```python
from build123d import *

# Parameters (mm, degrees)
BASE_FLANGE1_DEPTH           = 3.175
SKETCH8_W                    = 12.7
SKETCH8_H                    = 3.175
CUT_EXTRUDE2_DEPTH           = 309.926847379
SKETCH11_R                   = 3.175
CUT_EXTRUDE4_DEPTH           = 309.926847379
SKETCH21_R                   = 2.5527
CUT_EXTRUDE5_DEPTH           = 309.926847379
SKETCH23_W                   = 25.4
SKETCH23_H                   = 3.175
TAB1_DEPTH                   = 3.175
CSK_FOR_M3_SFHCS1_AT_2_COUNT = 2
CSK_FOR_M3_SFHCS1_AT_2_PITCH = 16
CSK_FOR_M3_SFHCS1_AT_3_COUNT = 2
CSK_FOR_M3_SFHCS1_AT_3_PITCH = 27.712812921
CSK_FOR_M3_SFHCS1_AT_4_COUNT = 2
CSK_FOR_M3_SFHCS1_AT_4_PITCH = 32
CSK_FOR_M3_SFHCS1_AT_5_COUNT = 2
CSK_FOR_M3_SFHCS1_AT_5_PITCH = 27.712812921
CSK_FOR_M3_SFHCS1_AT_6_COUNT = 2
CSK_FOR_M3_SFHCS1_AT_6_PITCH = 16


# Sheet-metal steps are written as plain solids
with BuildPart() as part:
    # Sketch1 → Base-Flange1 (new body)
    with BuildSketch(Plane(origin=(0, 0, 0), x_dir=(0, 0, -1), z_dir=(1, 0, 0))):
        with BuildLine():
            Line((0, -80.9625), (0, 80.9625))
            Line((0, 80.9625), (-110.597916699, 80.9625))
            ThreePointArc((-110.597916699, 80.9625), (-137.538685062, 85.883926782), (-160.999479175, 100.0125))
            ThreePointArc((-160.999479175, 100.0125), (-201.559524406, 89.942756121), (-177.8, 55.5625))
            Line((-177.8, 55.5625), (-25.4, 55.5625))
            Line((-25.4, 55.5625), (-25.4, -68.2625))
            Line((-25.4, -68.2625), (-279.4, -68.2625))
            Line((-279.4, -68.2625), (-279.4, -80.9625))
            Line((-279.4, -80.9625), (-44.45, -80.9625))
            Line((-44.45, -80.9625), (-44.45, -131.7625))
            Line((-44.45, -131.7625), (-34.925, -131.7625))
            Line((-34.925, -131.7625), (-34.925, -125.4125))
            Line((-34.925, -125.4125), (-38.1, -125.4125))
            Line((-38.1, -125.4125), (-38.1, -106.3625))
            Line((-38.1, -106.3625), (-6.35, -106.3625))
            Line((-6.35, -106.3625), (-6.35, -125.4125))
            Line((-6.35, -125.4125), (-9.525, -125.4125))
            Line((-9.525, -125.4125), (-9.525, -131.7625))
            Line((-9.525, -131.7625), (0, -131.7625))
            Line((0, -131.7625), (0, -80.9625))
        make_face()
    extrude(amount=-BASE_FLANGE1_DEPTH)

    # Sketch8 → Cut-Extrude2 (cut, through all)
    with BuildSketch(Plane(origin=(0, 0, 0), x_dir=(0, 0, -1), z_dir=(1, 0, 0))):
        with Locations((-19.05, -6.35)):
            Rectangle(SKETCH8_W, SKETCH8_H)
        with Locations((-19.05, -34.925)):
            Rectangle(SKETCH8_W, SKETCH8_H)
    extrude(amount=-CUT_EXTRUDE2_DEPTH, mode=Mode.SUBTRACT)

    # Sketch11 → Cut-Extrude4 (cut, through all)
    with BuildSketch(Plane(origin=(0, 0, 0), x_dir=(0, 0, -1), z_dir=(1, 0, 0))):
        with Locations((-177.8, 80.9625)):
            Circle(SKETCH11_R)
    extrude(amount=-CUT_EXTRUDE4_DEPTH, mode=Mode.SUBTRACT)

    # Sketch21 → Cut-Extrude5 (cut, through all)
    with BuildSketch(Plane(origin=(0, 0, 0), x_dir=(0, 0, -1), z_dir=(1, 0, 0))):
        with Locations((-38.1, -74.6125)):
            Circle(SKETCH21_R)
        with Locations((-110.066666667, -74.6125)):
            Circle(SKETCH21_R)
        with Locations((-182.033333333, -74.6125)):
            Circle(SKETCH21_R)
        with Locations((-254, -74.6125)):
            Circle(SKETCH21_R)
        with Locations((-12.7, 61.9125)):
            Circle(SKETCH21_R)
        with Locations((-38.1, 74.6125)):
            Circle(SKETCH21_R)
        with Locations((-63.5, 61.9125)):
            Circle(SKETCH21_R)
    extrude(amount=-CUT_EXTRUDE5_DEPTH, mode=Mode.SUBTRACT)

    # Sketch23 → Tab1 (add)
    with BuildSketch(Plane(origin=(0, 0, 0), x_dir=(0, 0, -1), z_dir=(1, 0, 0))):
        with Locations((-218.016666667, -66.675)):
            Rectangle(SKETCH23_W, SKETCH23_H)
        with Locations((-146.05, -66.675)):
            Rectangle(SKETCH23_W, SKETCH23_H)
        with Locations((-74.083333333, -66.675)):
            Rectangle(SKETCH23_W, SKETCH23_H)
    extrude(amount=-TAB1_DEPTH)

    # Sketch25 → CSK for M3 SFHCS1 (revolve, cut)
    with BuildSketch(Plane(origin=(0, 80.9625, 161.8), x_dir=(0, 0, -1), z_dir=(0, 1, 0))):
        Polygon((0, 0), (0, 3.175), (1.7, 3.175), (1.7, 1.66), (3.36, 0), align=None)
    csk_for_m3_sfhcs1 = revolve(axis=Axis((6.35, 80.9625, 161.8), (-1, 0, 0)), mode=Mode.SUBTRACT)

    # CSK for M3 SFHCS1 at 2: CSK for M3 SFHCS1 ×2
    with Locations(*[Vector(0, -0.8660254037844389, 0.4999999999999998) * (i * CSK_FOR_M3_SFHCS1_AT_2_PITCH) for i in range(1, CSK_FOR_M3_SFHCS1_AT_2_COUNT)]):
        add(csk_for_m3_sfhcs1, mode=Mode.SUBTRACT)

    # CSK for M3 SFHCS1 at 3: CSK for M3 SFHCS1 ×2
    with Locations(*[Vector(0, -0.500000000000002, 0.8660254037844376) * (i * CSK_FOR_M3_SFHCS1_AT_3_PITCH) for i in range(1, CSK_FOR_M3_SFHCS1_AT_3_COUNT)]):
        add(csk_for_m3_sfhcs1, mode=Mode.SUBTRACT)

    # CSK for M3 SFHCS1 at 4: CSK for M3 SFHCS1 ×2
    with Locations(*[(0, 0, i * CSK_FOR_M3_SFHCS1_AT_4_PITCH) for i in range(1, CSK_FOR_M3_SFHCS1_AT_4_COUNT)]):
        add(csk_for_m3_sfhcs1, mode=Mode.SUBTRACT)

    # CSK for M3 SFHCS1 at 5: CSK for M3 SFHCS1 ×2
    with Locations(*[Vector(0, 0.5000000000000007, 0.8660254037844384) * (i * CSK_FOR_M3_SFHCS1_AT_5_PITCH) for i in range(1, CSK_FOR_M3_SFHCS1_AT_5_COUNT)]):
        add(csk_for_m3_sfhcs1, mode=Mode.SUBTRACT)

    # CSK for M3 SFHCS1 at 6: CSK for M3 SFHCS1 ×2
    with Locations(*[Vector(0, 0.8660254037844379, 0.5000000000000013) * (i * CSK_FOR_M3_SFHCS1_AT_6_PITCH) for i in range(1, CSK_FOR_M3_SFHCS1_AT_6_COUNT)]):
        add(csk_for_m3_sfhcs1, mode=Mode.SUBTRACT)


solid = part.part
```
Geometry: final body of the model. Coordinates: model frame, mm. Give positions to 0.01 mm unless a question says otherwise; leave off trailing zeros. Order: outer loops, then holes, each group sorted by start corner. A loop starts at its lowest first (then second) coordinate and runs counter-clockwise, first axis right, second up. Notation, with made-up numbers: (17.5, 85.5) -> (48.5, 85.5) arc R18 cw to (48.5, 116.5) -> close; hole circle Ø8 at (-9.5, 26.25). An arc over 180 degrees is marked (long way). Write each question's results on one line, items separated by ' | '. Start each with the question number.
1) Section D-D (x = -0.75). Count the separate pieces of the cut face and the enclosed holes in it, then the cut area to 3 significant figures.
2) Draft query along Y for faces 1 (the cylindrical face through (-1.565, 77.863, 178.488)), 2 (the flat face through (-3.175, 58, 89)), 3 (the cylindrical face through (-1.57, 85.75, 137.18)), 4 (the cylindrical face through (-1.6, 90.6, 201.3)). Return one class per face: pulls with the +Y half, pulls with the -Y half, needs draft (parallel to the pull), parting line crosses it, or undercut.
3) Line query: line 1 (Y direction, x = -2, z = 25); line 2 (Z direction, x = -2, y = 96); line 3 (Y direction, x = -2.75, z = 46.5). Output: solid intervals per line, ascending. Write a range as from..to.
4) First-contact query: pin 1 (1 mm diameter, centred on x = -1, z = 7.5, fed in from +Y); pin 2 (1 mm diameter, centred on x = -2, z = 178.5, fed in from -Y); pin 3 (5.5 mm diameter, centred on y = 94.82, z = 185.8, fed in from +X). Flat tips, straight axial feed; report the tip coordinate or a pass-through.
5) Section C-C (z = 217.5). Return loops of the section in (x, y) (1 decimal).
6) Section B-B (y = -100.5). Return loops of the section in (x, z) (3 decimals), then the cut area to 3 significant figures.
7) Section A-A (z = 93.5). Return loops of the section in (x, y) (1 decimal), then the cut area to 3 significant figures.
Calculated:
1) separate pieces: 1 | enclosed holes: 14 | area: 14,300 mm2
2) face 1: undercut | face 2: needs draft | face 3: pulls with the +Y half | face 4: undercut
3) line 1: -106.36..-36.51, -33.34..-7.94, -4.76..80.96 | line 2: 156.05..168.58, 171.02..184.58, 187.02..198.27 | line 3: -80.96..-68.26, 55.56..80.96
4) pin 1: y = 80.96 | pin 2: y = -80.96 | pin 3: x = -0.61
5) outline: (-3.2, -81) -> (0, -81) -> (0, -65.1) -> (-3.2, -65.1) -> close
6) outline: (-3.175, 0) -> (0, 0) -> (0, 44.45) -> (-3.175, 44.45) -> close | area: 141 mm2
7) outline: (-3.2, -81) -> (0, -81) -> (0, -68.3) -> (-3.2, -68.3) -> close; (-3.2, 55.6) -> (0, 55.6) -> (0, 81) -> (-3.2, 81) -> close | area: 121 mm2
